from build123d import *

# Parameters (mm, degrees)
SKETCH_R            = 6.5
PAD_DEPTH           = 10
POCKET_DEPTH        = 12
LINEARPATTERN_COUNT = 7
LINEARPATTERN_PITCH = 21.666667


with BuildPart() as part:
    # Sketch → Pad (new body)
    with BuildSketch(Plane.XY):
        with BuildLine():
            ThreePointArc((-15, 0), (0, -15), (15, 0))
            Line((15, 0), (15, 170))
            ThreePointArc((15, 170), (0, 185), (-15, 170))
            Line((-15, 170), (-15, 0))
        make_face()
        Circle(SKETCH_R, mode=Mode.SUBTRACT)
        with Locations((0, 170)):
            Circle(SKETCH_R, mode=Mode.SUBTRACT)
    extrude(amount=PAD_DEPTH)

    # Sketch001 (on Face8 of Pad) → Pocket (cut)
    with BuildSketch(Plane.XY.offset(10)):
        with BuildLine():
            ThreePointArc((12, 26), (10, 28), (8, 26))
            Line((8, 26), (8, 14))
            ThreePointArc((8, 14), (10, 12), (12, 14))
            Line((12, 14), (12, 26))
        make_face()
    pocket = extrude(amount=-POCKET_DEPTH, mode=Mode.SUBTRACT)

    # LinearPattern: Pocket ×7
    with Locations(*[(0, i * LINEARPATTERN_PITCH, 0) for i in range(1, LINEARPATTERN_COUNT)]):
        add(pocket, mode=Mode.SUBTRACT)


solid = part.part
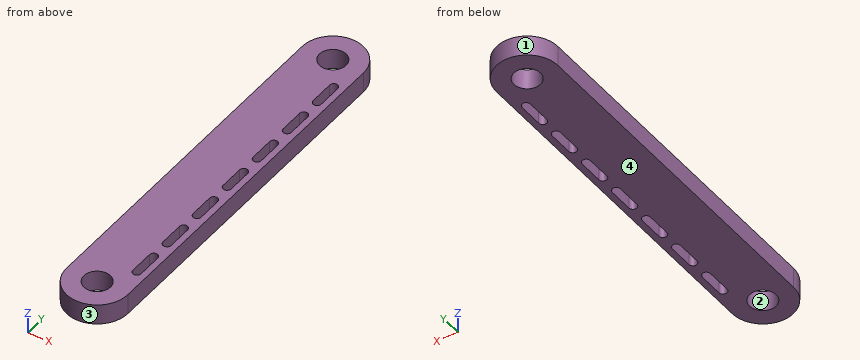
Source: CAD feature listing. Evaluate the final solid. Frame: model axes, mm. Face numbers are marked on the shaded views. Coordinates: 2 decimals unless noted, no trailing zeros. Loops run counter-clockwise (first coordinate to the right, second up) from the corner with the lowest first, then second, coordinate; pieces in that order, holes last. Notation, with made-up numbers: (4.25, 0) - (56.25, 0) arc R11 ccw to (56.25, 4) - close; hole circle Ø2 at (45, -37.75). An arc over 180 degrees is marked (long way). One line per item, written item: value. Start each with the question number.
1. Ray query, L1, parallel to Y at x = 0, z = 2.25; L2, parallel to X at y = 154.5, z = 7.25; L3, parallel to Y at x = -2.5, z = 3.75. Return the intervals inside material, ascending.
2. Mould query, pull axis Y, two halves, no side actions, for the marked faces 1, 2, 3 and 4. Classes: pulls with the +Y half, pulls with the -Y half, needs draft (parallel to the pull), parting line crosses it, or undercut.
3. Contact query for flat-ended pins moving along their axis: P1, Ø2, axis at x = -6, z = 7, coming from the -Y side; P2, Ø8, axis at x = 0, y = 0, coming from the -Z side (3 decimals). Output: stop coordinate, or through.
4. Section C-C (z = 5). State how many separate pieces and enclosed holes the cut face has, and give its area (3 significant figures).
5. Section A-A (x = 0). Return the cut outline in (y, z), and give its area (3 significant figures).
6. Section B-B (y = 17.5). Return the cut outline in (x, z), and give its area (3 significant figures).
Verdict:
1. L1: y = -15 to -6.5, 6.5 to 163.5, 176.5 to 185
1. L2: x = -15 to 8, 12 to 15
1. L3: y = -14.79 to -6, 6 to 164, 176 to 184.79
2. face 1: pulls with the +Y half
2. face 2: undercut
2. face 3: pulls with the -Y half
2. face 4: needs draft
3. P1: stops at y = -14.14
3. P2: passes through
4. separate pieces: 1
4. enclosed holes: 9
4. area: 5,120 mm2
5. outline: (-15, 0) - (-6.5, 0) - (-6.5, 10) - (-15, 10) - close; (6.5, 0) - (163.5, 0) - (163.5, 10) - (6.5, 10) - close; (176.5, 0) - (185, 0) - (185, 10) - (176.5, 10) - close
5. area: 1,740 mm2
6. outline: (-15, 0) - (8, 0) - (8, 10) - (-15, 10) - close; (12, 0) - (15, 0) - (15, 10) - (12, 10) - close
6. area: 260 mm2
